```python
from build123d import *

# Parameters (mm, degrees)
EXTRUDE_THIN1_DEPTH                                  = 35
CUT_EXTRUDE1_REACH                                   = 39.527
SKETCH2_R                                            = 1.55575
CSK_FOR_M1_6_COUNTERSUNK_FLAT_HEAD_SCREW_D           = 1.8
CSK_FOR_M1_6_COUNTERSUNK_FLAT_HEAD_SCREW_DEPTH       = 119
CSK_FOR_M1_6_COUNTERSUNK_FLAT_HEAD_SCREW_CSINK_D     = 3.6
CSK_FOR_M1_6_COUNTERSUNK_FLAT_HEAD_SCREW_CSINK_ANGLE = 90
CSK_FOR_M1_6_COUNTERSUNK_FLAT_HEAD_SCREW_TIP         = 0.540774557


with BuildPart() as part:
    # Sketch1 → Extrude-Thin1 (new body)
    with BuildSketch(Plane.XY):
        with BuildLine():
            Line((-12.5, 6.2), (-12.5, 1))
            ThreePointArc((-12.5, 1), (-12.207106781, 0.292893219), (-11.5, 0))
            Line((-11.5, 0), (11.5, 0))
            ThreePointArc((11.5, 0), (12.207106781, 0.292893219), (12.5, 1))
            Line((12.5, 1), (12.5, 6.2))
            Line((12.5, 6.2), (11.5, 6.2))
            Line((11.5, 6.2), (11.5, 1))
            Line((11.5, 1), (-11.5, 1))
            Line((-11.5, 1), (-11.5, 6.2))
            Line((-11.5, 6.2), (-12.5, 6.2))
        make_face()
    extrude(amount=EXTRUDE_THIN1_DEPTH)

    # Sketch2 → Cut-Extrude1 (cut, up to next)
    with BuildSketch(Plane(origin=(0, 1, 0), x_dir=(1, 0, 0), z_dir=(0, 1, 0)), mode=Mode.PRIVATE) as cut_extrude1_sk1:
        with Locations(Location((0, -17.5, 0), (0, 0, 180))):
            Circle(SKETCH2_R)
    cut_extrude1_tool1 = extrude(cut_extrude1_sk1.sketch, amount=-CUT_EXTRUDE1_REACH, mode=Mode.PRIVATE) & part.part
    add(cut_extrude1_tool1.solids().sort_by_distance((0, 1, 17.5))[0], mode=Mode.SUBTRACT)

    # CSK for M1.6 Countersunk Flat Head Screw1
    with Locations(Plane(origin=(5.666541612, 1, 11.833458388), x_dir=(1, 0, 0), z_dir=(0, 1, 0))):
        with Locations((0, 0), (1.005788686, -12.33887191), (-11.333083224, -11.333083224), (-12.33887191, 1.005788686)):
            CounterSinkHole(CSK_FOR_M1_6_COUNTERSUNK_FLAT_HEAD_SCREW_D / 2, CSK_FOR_M1_6_COUNTERSUNK_FLAT_HEAD_SCREW_CSINK_D / 2, depth=CSK_FOR_M1_6_COUNTERSUNK_FLAT_HEAD_SCREW_DEPTH, counter_sink_angle=CSK_FOR_M1_6_COUNTERSUNK_FLAT_HEAD_SCREW_CSINK_ANGLE)
            with Locations((0, 0, -(CSK_FOR_M1_6_COUNTERSUNK_FLAT_HEAD_SCREW_DEPTH + CSK_FOR_M1_6_COUNTERSUNK_FLAT_HEAD_SCREW_TIP / 2))):  # 118° drill point
                Cone(0, CSK_FOR_M1_6_COUNTERSUNK_FLAT_HEAD_SCREW_D / 2, CSK_FOR_M1_6_COUNTERSUNK_FLAT_HEAD_SCREW_TIP, mode=Mode.SUBTRACT)


solid = part.part
```
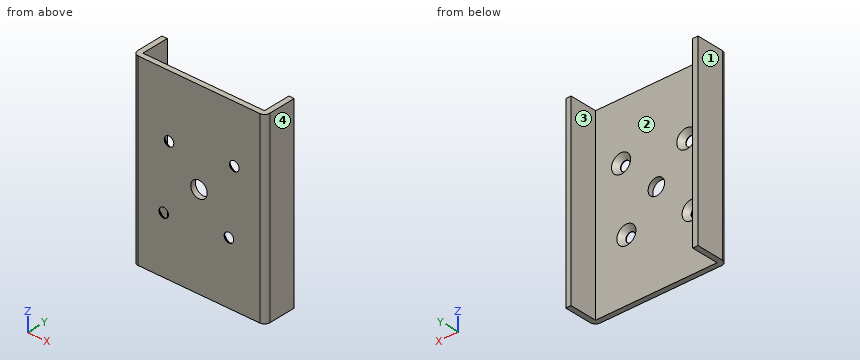
Geometry: final body of the model. Coordinates: model frame, mm. Face numbers are marked on the shaded views. Give positions to 0.01 mm unless a question says otherwise; leave off trailing zeros. Write each loop counter-clockwise with the first axis right and the second up, starting at its lowest first coordinate (ties: lowest second). Pieces come first, ordered by that corner, then holes.
1. Draft query along X for the marked faces 1, 2, 3 and 4. Return one class per face: released by +X, released by -X, zero draft, split by the parting line, or undercut.
2. Section query D-D, the plane z = 30.5. Return loops of the section in (x, y).
3. Section query B-B, the plane x = 0. Return loops of the section in (y, z), then the cut area to 3 significant figures.
4. Section query A-A, the plane z = 17.5. Return loops of the section in (x, y), then the cut area to 3 significant figures.
5. Line query: probe 1 along X at (y, z) = (5.5, 8); probe 2 along Z at (x, y) = (-5.75, 0.5); probe 3 along Z at (x, y) = (0, 0.5). Output: solid intervals per line, ascending.
6. Section query C-C, the plane y = 2.75. Return loops of the section in (x, z).
7. Pin query (flat end, axial travel): P1, Ø4, axis at x = -3, z = 8.5, coming from the -Y side; P2, Ø2.5, axis at x = 0, z = 17.5, coming from the -Y side; P3, Ø2.5, axis at x = 6.67, z = 24.17, coming from the +Y side; P4, Ø2, axis at x = -5.67, z = 23.17, coming from the +Y side. Return the tip coordinate at first contact, or that it passes through.
Computed:
1. face 1: released by -X
1. face 2: undercut
1. face 3: undercut
1. face 4: released by +X
2. outline: (-12.5, 1) arc R1 ccw to (-11.5, 0) - (11.5, 0) arc R1 ccw to (12.5, 1) - (12.5, 6.2) - (11.5, 6.2) - (11.5, 1) - (-11.5, 1) - (-11.5, 6.2) - (-12.5, 6.2) - close
3. outline: (0, 0) - (1, 0) - (1, 15.94) - (0, 15.94) - close; (0, 19.06) - (1, 19.06) - (1, 35) - (0, 35) - close
3. area: 31.9 mm2
4. outline: (-12.5, 1) arc R1 ccw to (-11.5, 0) - (-1.56, 0) - (-1.56, 1) - (-11.5, 1) - (-11.5, 6.2) - (-12.5, 6.2) - close; (1.56, 0) - (11.5, 0) arc R1 ccw to (12.5, 1) - (12.5, 6.2) - (11.5, 6.2) - (11.5, 1) - (1.56, 1) - close
4. area: 31.9 mm2
5. probe 1: x = -12.5 to -11.5, 11.5 to 12.5
5. probe 2: z = 0 to 9.91, 11.74 to 21.87, 24.46 to 35
5. probe 3: z = 0 to 15.94, 19.06 to 35
6. outline: (-12.5, 0) - (-11.5, 0) - (-11.5, 35) - (-12.5, 35) - close; (11.5, 0) - (12.5, 0) - (12.5, 35) - (11.5, 35) - close
7. P1: stops at y = 0
7. P2: passes through
7. P3: stops at y = 0.45
7. P4: stops at y = 0.2
